Autodesk Inventor part; units mm, degrees
ref_plane "YZ Plane" through (0, 0, 0) normal (1, 0, 0) x (0, 1, 0)
ref_plane "XZ Plane" through (0, 0, 0) normal (0, 1, 0) x (-1, 0, 0)
ref_plane "XY Plane" through (0, 0, 0) normal (0, 0, 1) x (1, 0, 0)
sketch "Sketch1" plane through (0, 0, 0) normal (0, 1, 0) x (-1, 0, 0)
  line L0 (8.45, 6.25) -> (-8.45, 6.25)
  line L1 (-10.45, 4.25) -> (-10.45, -4.25)
  line L2 (-8.45, -6.25) -> (8.45, -6.25)
  line L3 (10.45, -4.25) -> (10.45, 4.25)
  line L4 (10.45, 6.25) -> (-10.45, -6.25) construction
  line L5 (-10.45, 6.25) -> (10.45, -6.25) construction
  line L6 (8.45, -6.25) -> (10.45, -4.25)
  line L7 (10.45, 4.25) -> (8.45, 6.25)
  line L8 (-8.45, 6.25) -> (-10.45, 4.25)
  line L9 (-10.45, -4.25) -> (-8.45, -6.25)
  point P0 (0, 0)
  dimension "d0" = 20.9
  dimension "d1" = 12.5
  dimension "d2" = 2
  dimension "d3" = 2
extrude "Extrusion1" add sketch "Sketch1" along normal mid plane 1.7
equation "\"d0\" = CMWidth"
equation "\"d1\" = CMLength"
equation "\"d2\" = CMChamfer"
equation "\"d3\" = d2"
properties part number "ControlMarker_Single" material "Paper"
Work out the finished part from the listing and answer in its coordinate system (mm). Round coordinates to 2 decimals unless told otherwise and drop trailing zeros. Loops run counter-clockwise (first coordinate to the right, second up) from the corner with the lowest first, then second, coordinate; pieces in that order, holes last.
(1) The part is cut by section B-B, the plane z = -4.5. Give the vertices of the cut face in (x, y).
Computed values:
outline: (-10.2, -0.85) - (10.2, -0.85) - (10.2, 0.85) - (-10.2, 0.85) - close
(2) Find the intervals of material crossed by L1, parallel to X at y = 0.2, z = 5; L2, parallel to X at y = -0.45, z = -5.25; L3, parallel to Z at x = 9.25, y = -0.05, in increasing order.
Computed values:
L1: x = -9.7 to 9.7
L2: x = -9.45 to 9.45
L3: z = -5.45 to 5.45
(3) The part is cut by section C-C, the plane x = 9. Give the vertices of the cut face in (y, z).
Computed values:
outline: (-0.85, -5.7) - (0.85, -5.7) - (0.85, 5.7) - (-0.85, 5.7) - close
(4) The part is cut by section A-A, the plane y = -0.45. Give the vertices of the cut face in (x, z), and give its area (3 significant figures).
Computed values:
outline: (-10.45, -4.25) - (-8.45, -6.25) - (8.45, -6.25) - (10.45, -4.25) - (10.45, 4.25) - (8.45, 6.25) - (-8.45, 6.25) - (-10.45, 4.25) - close
area: 253 mm2
